Input: part model. Units: mm. Frame: model coordinates. A direction names the side the tool comes from. Give positions to 0.01 mm unless a question says otherwise; leave off trailing zeros. Loops run counter-clockwise (first coordinate to the right, second up) from the corner with the lowest first, then second, coordinate; pieces in that order, holes last. Notation, with made-up numbers: M 39.25,67.25 L 85.25,67.25 A22 cw 85.25,104.25 Z; hole C 28,44 d4. An arc over 180 degrees is marked long. One line per item, written item: value. Start each with the question number.
(1) Section C-C on x = 6.5. Output: boundary loops of the cut face in (y, z).
(2) Pin query (flat end, axial travel): P1, Ø2, axis at x = -5, z = 2.5, coming from the +Y side; P2, Ø2, axis at x = 7.5, z = 6.5, coming from the -Y side; P3, Ø2.5, axis at x = 13.5, z = 7, coming from the -Y side; P4, Ø5, axis at x = 4.5, y = -7, coming from the -Z side. Return the tip coordinate at first contact, or that it passes through.
(3) Access query for faces 5 (the flat face through (11.1, 28, 2)), 6 (the flat face through (15, 28, 4.8)), 7 (the flat face through (-15, -27.5, 6)), 8 (the flat face through (2.725, 22, 4)). Directions: +Z, -Z, +X, -X, +Y, -Y. A direction counts if a zero-diameter tool reaches every point of the face in a straight line with its end or side. Return the directions, or none.
(4) Section B-B on z = 6.75. Output: boundary loops of the cut face in (x, y) (3 decimals), plus the area to 3 significant figures.
(5) Ray query, line 1 along X through (y, z) = (-23.5, 2.4); line 2 along Z through (x, y) = (-14.5, -22); line 3 along X through (y, z) = (-26.75, 2.4). Return the intervals inside material, ascending. Write a range as from..to.
(6) Pull-direction query (X, two-part tool) for faces 1 (the cylindrical face through (13.26, -23.42, 2.56)), 2 (the flat face through (17.9, 0, 4)), 3 (the flat face through (15, 27.5, 6)), 4 (the flat face through (-11.1, -28, 2)); classes: released by +X, released by -X, zero draft, split by the parting line, or undercut.
(7) Section A-A on x = -9.6. Output: boundary loops of the cut face in (y, z).
Solid Edge part; units mm, degrees
sketch "Sketch1" plane through (0, 0, 0) normal (0, 0, 1) x (1, 0, 0)
  line L0 (-17.9, -27.5) -> (17.9, -27.5)
  line L1 (17.9, -27.5) -> (17.9, 27.5)
  line L2 (17.9, 27.5) -> (-17.9, 27.5)
  line L3 (-17.9, 27.5) -> (-17.9, -27.5)
extrude "Protrusion1" add sketch "Sketch1" along normal blind 8
sketch "Sketch2" plane through (0, -27.5, 4) normal (0, -1, 0) x (1, 0, 0)
  line L0 (-11.1, 0.8) -> (-17.9, 0.8)
  line L1 (-17.9, 0.8) -> (-17.9, -4)
  line L2 (-17.9, -4) -> (-11.1, -4)
  line L3 (-11.1, -4) -> (-11.1, 0.8)
  line L4 (11.1, 0.8) -> (17.9, 0.8)
  line L5 (17.9, 0.8) -> (17.9, -4)
  line L6 (17.9, -4) -> (11.1, -4)
  line L7 (11.1, -4) -> (11.1, 0.8)
extrude "ExtrudedProtrusion_2" add sketch "Sketch2" along normal blind 2
sketch "Sketch3" plane through (0, 27.5, 4) normal (0, 1, 0) x (-1, 0, 0)
  line L0 (-17.9, 0.8) -> (-11.1, 0.8)
  line L1 (-11.1, 0.8) -> (-11.1, -4)
  line L2 (-11.1, -4) -> (-17.9, -4)
  line L3 (-17.9, -4) -> (-17.9, 0.8)
  line L4 (11.1, 0.8) -> (17.9, 0.8)
  line L5 (17.9, 0.8) -> (17.9, -4)
  line L6 (17.9, -4) -> (11.1, -4)
  line L7 (11.1, -4) -> (11.1, 0.8)
extrude "ExtrudedProtrusion_3" add sketch "Sketch3" along normal blind 2
hole "Hole_3" at (-14.5, -29.5, 2.4) direction (0, 1, 0) diameter 2.5 depth 12 tip angle 118
hole "Hole1" at (14.5, -29.5, 2.4) direction (0, 1, 0) diameter 2.5 depth 12 tip angle 118
sketch "Sketch4" plane through (0, 0, 8) normal (0, 0, 1) x (0, -1, 0)
  line L0 (26.5, 0) -> (26.5, -8.482)
  arc A0 (26.5, -8.482) -> (27.5, -11.1) centre (27.5, -9.6) ccw
  line L1 (27.5, 11.1) -> (27.5, -11.1)
  arc A1 (27.5, 11.1) -> (26.5, 8.482) centre (27.5, 9.6) ccw
  line L2 (26.5, 0) -> (26.5, 8.482)
  arc A2 (-27.5, -8.1) -> (-27.5, -11.1) centre (-27.5, -9.6) cw
  line L3 (-27.5, -11.1) -> (-27.5, -8.1)
  arc A3 (-27.5, 11.1) -> (-27.5, 8.1) centre (-27.5, 9.6) cw
  line L4 (-27.5, 11.1) -> (-27.5, 8.1)
extrude "ExtrudedCutout_1" cut sketch "Sketch4" against normal blind 8
sketch "Sketch5" plane through (0, 0, 8) normal (0, 0, 1) x (1, 0, 0)
  arc A0 (1.6, 24.4524) -> (2.725, 23) centre (1.225, 23) cw
  line L0 (2.725, 23) -> (2.725, 21.5)
  arc A1 (2.725, 21.5) -> (1.5998, 20.0476) centre (1.225, 21.5) cw
  arc A2 (1.5998, 20.0476) -> (-1.5998, 20.0476) centre (0, 20.0254) cw
  arc A3 (-2.725, 21.5) -> (-1.5998, 20.0476) centre (-1.225, 21.5) ccw
  line L1 (-2.725, 23) -> (-2.725, 21.5)
  arc A4 (-1.5998, 24.4524) -> (-2.725, 23) centre (-1.225, 23) ccw
  line L2 (-1.5998, 27.5) -> (-1.5998, 24.4524)
  line L3 (0, 27.5) -> (-1.5998, 27.5)
  line L4 (0, 27.5) -> (1.6, 27.5)
  line L5 (1.6, 27.5) -> (1.6, 24.4524)
extrude "Cutout1" cut sketch "Sketch5" against normal up to next
properties material "Polycarbonate"
Output values:
1. outline: M -26.5,0 L 27.5,0 L 27.5,8 L -26.5,8 Z
2. P1: stops at y = 27.5
2. P2: stops at y = -26.5
2. P3: stops at y = -27.5
2. P4: stops at z = 0
3. face 5: +Z, -Z, +Y
3. face 6: +Z, +X, -X, +Y
3. face 7: +Z, +X, -X, -Y
3. face 8: +Z, -Z
4. outline: M -17.9,-27.5 L -11.1,-27.5 A1.5 cw -8.482,-26.5 L 0,-26.5 L 8.482,-26.5 A1.5 cw 11.1,-27.5 L 17.9,-27.5 L 17.9,27.5 L 11.1,27.5 A1.5 cw 8.1,27.5 L 1.6,27.5 L 1.6,24.452 A1.5 cw 2.725,23 L 2.725,21.5 A1.5 cw 1.6,20.048 A1.6 cw long -1.6,20.048 A1.5 cw -2.725,21.5 L -2.725,23 A1.5 cw -1.6,24.452 L -1.6,27.5 L -8.1,27.5 A1.5 cw -11.1,27.5 L -17.9,27.5 Z
4. area: 1,900 mm²
5. line 1: x = -17.9..-15.75, -13.25..13.25, 15.75..17.9
5. line 2: z = 0..1.15, 3.65..8
5. line 3: x = -17.9..-15.75, -13.25..-10.9, 10.9..13.25, 15.75..17.9
6. face 1: undercut
6. face 2: released by +X
6. face 3: zero draft
6. face 4: undercut
7. outline: M -26,0 L 26,0 L 26,8 L -26,8 Z
